Can you work these out from the model? Positions are in its coordinate system, mm. Round coordinates to 2 decimals unless told otherwise and drop trailing zeros. Loops run counter-clockwise (first coordinate to the right, second up) from the corner with the lowest first, then second, coordinate; pieces in that order, holes last. Notation, with made-up numbers: (26, -20.5) -> (44, -20.5) arc R34 cw to (44, 11.5) -> close; hole circle Ø8 at (16.5, 33.25). An arc over 180 degrees is marked (long way). Write each question's results on one line, items separated by ' | '.
from build123d import *

# Parameters (mm, degrees)
SKETCH1_R           = 25
BOSS_EXTRUDE1_DEPTH = 135


with BuildPart() as part:
    # Sketch1 → Boss-Extrude1 (new body)
    with BuildSketch(Plane(origin=(0, 0, 0), x_dir=(0, 0, -1), z_dir=(1, 0, 0))):
        Circle(SKETCH1_R)
    boss_extrude1 = extrude(amount=BOSS_EXTRUDE1_DEPTH)

    # Sketch3 → Revolve1 (revolve)
    with BuildSketch(Plane.XY, mode=Mode.PRIVATE) as revolve1_sk:
        with BuildLine():
            Line((0, 0), (-45.458392513, 0))
            add(Edge.make_bspline(
                [(-45.458392513, 0), (-45.458392513, 20.183781855), (-30.991238831, 40), (0, 40)],
                knots=[0, 0, 0, 0, 1, 1, 1, 1], degree=3))
            Line((0, 40), (0, 0))
        make_face()
    revolve1 = revolve(revolve1_sk.sketch.rotate(Axis((-100.078673334, 0, 0), (1, 0, 0)), 90), axis=Axis((-100.078673334, 0, 0), (1, 0, 0)))

    # Mirror1: Boss-Extrude1, Revolve1 across plane
    add(boss_extrude1.mirror(Plane(origin=(135, 0, 0), x_dir=(0, 0, 1), z_dir=(1, 0, 0))))
    add(revolve1.mirror(Plane(origin=(135, 0, 0), x_dir=(0, 0, 1), z_dir=(1, 0, 0))))


solid = part.part
1. Please list where these lines run through material, in increasing order: line 1 (X direction, y = -23.5, z = -10); line 2 (X direction, y = 29.5, z = -14); line 3 (Y direction, x = 198, z = 13). Write a range as from..to.
Final values:
line 1: -36.24..0, 270..306.24 | line 2: -28.02..0, 270..298.02 | line 3: -21.35..21.35
2. If we section it at A-A (x = 125.5): List the corners of the cut face in (y, z) for me.
Final values:
outline: circle Ø50 at (0, 0)
3. Will these pins go through, and if not, where does the flat tip stop? pin 1 (4 mm diameter, centred on x = 161, z = 4.5, fed in from -Y); pin 2 (8 mm diameter, centred on x = 185, y = -11.5, fed in from -Z); pin 3 (8 mm diameter, centred on x = 112.5, z = -30.5, fed in from -Y); pin 4 (24 mm diameter, centred on y = -18.5, z = -11.5, fed in from +X).
Final values:
pin 1: y = -24.87 | pin 2: z = -23.85 | pin 3: through | pin 4: x = 314.29
4. We'd pull the mould along X, two halves only. Please class faces 1 (the face through (270, -18.34, 17.22)), 2 (the face through (0, -18.34, 17.22)): pulls with the +X half, pulls with the -X half, needs draft (parallel to the pull), parting line crosses it, or undercut.
Final values:
face 1: undercut | face 2: undercut
